Autodesk Inventor part; units mm, degrees
ref_plane "YZ Plane" through (0, 0, 0) normal (1, 0, 0) x (0, 1, 0)
ref_plane "XZ Plane" through (0, 0, 0) normal (0, 1, 0) x (-1, 0, 0)
ref_plane "XY Plane" through (0, 0, 0) normal (0, 0, 1) x (1, 0, 0)
sketch "Sketch1" plane through (0, 0, 0) normal (0, 1, 0) x (-1, 0, 0)
  line L0 (40.005, 40.005) -> (-40.005, 40.005)
  line L1 (-40.005, 40.005) -> (-40.005, -40.005)
  line L2 (-40.005, -40.005) -> (-33.3375, -40.005)
  line L3 (40.005, -40.005) -> (40.005, 40.005)
  line L4 (40.005, 40.005) -> (-40.005, -40.005) construction
  line L5 (-40.005, 40.005) -> (40.005, -40.005) construction
  line L6 (46.101, 46.101) -> (-46.101, 46.101)
  line L7 (-46.101, 46.101) -> (-46.101, -46.101)
  line L8 (-46.101, -46.101) -> (-33.3375, -46.101)
  line L9 (46.101, -46.101) -> (46.101, 46.101)
  line L10 (46.101, 46.101) -> (-46.101, -46.101) construction
  line L11 (-46.101, 46.101) -> (46.101, -46.101) construction
  line L12 (33.3375, -40.005) -> (33.3375, -46.101)
  line L13 (13.335, -40.005) -> (13.335, -46.101)
  line L14 (13.335, -40.005) -> (33.3375, -40.005)
  line L15 (33.3375, -46.101) -> (46.101, -46.101)
  line L16 (13.335, -46.101) -> (33.3375, -46.101)
  line L17 (33.3375, -40.005) -> (40.005, -40.005)
  line L18 (-20.9635, 41.5612) -> (22.9239, 41.5612) construction
  line L19 (22.9239, 41.5612) -> (22.9239, 28.3672) construction
  line L20 (22.9239, 28.3672) -> (-20.9635, 28.3672) construction
  line L21 (-20.9635, 28.3672) -> (-20.9635, 41.5612) construction
  line L22 (4.0005, -46.101) -> (4.0005, -40.005)
  line L23 (-4.0005, -46.101) -> (-4.0005, -40.005)
  line L24 (-13.335, -46.101) -> (-13.335, -40.005)
  line L25 (-33.3375, -46.101) -> (-33.3375, -40.005)
  line L26 (4.0005, -40.005) -> (13.335, -40.005)
  line L27 (-4.0005, -40.005) -> (4.0005, -40.005)
  line L28 (-4.0005, -46.101) -> (4.0005, -46.101)
  line L29 (4.0005, -46.101) -> (13.335, -46.101)
  line L30 (-13.335, -46.101) -> (-4.0005, -46.101)
  line L31 (-33.3375, -46.101) -> (-13.335, -46.101)
  line L32 (-33.3375, -40.005) -> (-13.335, -40.005)
  line L33 (-13.335, -40.005) -> (-4.0005, -40.005)
  point P0 (0, 0)
  dimension "baseLength" = 80.01
  dimension "d1" = 80.01
  dimension "d2" = 6.096
  dimension "toothLength" = 20.0025
  dimension "toothOffset" = 13.335
  dimension "d16" = 8.001
  dimension "d17" = 4.0005
  dimension "d18" = 20.0025
  dimension "d19" = 13.335
extrude "Extrusion1" add sketch "Sketch1" along normal blind 6.096 contours L3 L17 L14 L26 L27 L33 L32 L2 L1 L0
extrude "Extrusion2" add sketch "Sketch1" along normal blind 6.096 contours L12 L16 L13 L14 | L32 L24 L31 L25 | L22 L28 L23 L27
pattern_circular "Circular Pattern1" count 4 over 360 about axis through (0, -10, 0) along (0, 1, 0) of "Extrusion2"
equation "\"baseLength\" = glassLength"
equation "\"d1\" = baseLength"
equation "\"d2\" = woodThickness"
equation "\"toothLength\" = 0.25 * baseLength"
equation "\"d16\" = 0.4 * toothLength"
equation "\"d18\" = toothLength"
equation "\"d6\" = woodThickness"
equation "\"d8\" = woodThickness"
equation "\"woodThickness\" = 6.096"
equation "\"glassLength\" = 80.01"
equation "\"glassHeight\" = 80.772"
equation "\"lip\" = 9.525"
equation "\"lasorTol\" = 0.0635"
properties part number "CandleHolder-1"
Model file for the job. Use its own axes, mm. A direction names the side the tool comes from. Round coordinates to 2 decimals unless told otherwise and drop trailing zeros. Order: outer loops, then holes, each group sorted by start corner. A loop starts at its lowest first (then second) coordinate and runs counter-clockwise, first axis right, second up. Notation, with made-up numbers: (26.5, -2.5) -> (68.5, -2.5) arc R13 ccw to (68.5, 14.5) -> close; hole circle Ø8 at (22, 73). An arc over 180 degrees is marked (long way). Use one line per item in the form item = value.
Item 1: Cut at A-A, the plane z = 11. Write the cut outline in (x, y) (3 decimals).
Returned:
outline = (-40.005, 0) -> (40.005, 0) -> (40.005, 6.096) -> (-40.005, 6.096) -> close
Item 2: Tool access for faces 5 (the face through (43, 3, -13.335)), 6 (the face through (13.335, 3, -43)), 7 (the face through (37, 3, 40.005)): list every direction of +Z, -Z, +X, -X, +Y, -Y with a clear straight run to the whole face (end or side of a thin tool).
Returned:
face_5 = +X, +Y, -Y
face_6 = -Z, +Y, -Y
face_7 = +Z, +X, +Y, -Y
Item 3: Cut at B-B, the plane x = 37.5. Write the cut outline in (y, z) (3 decimals), and give its area (3 significant figures).
Returned:
outline = (0, -40.005) -> (6.096, -40.005) -> (6.096, 40.005) -> (0, 40.005) -> close
area = 488 mm^2
Item 4: Drill centre lines: line 1 (X direction, y = 4.75, z = 42.5) (1 decimal); line 2 (X direction, y = 2, z = 10.5) (3 decimals). Where is each one in solid material? Low to high.
Returned:
line_1 = -33.3 to -13.3, -4 to 4, 13.3 to 33.3
line_2 = -40.005 to 40.005
Item 5: Pull direction X, two halves, no side cores. Call faces 1 (the face through (33.338, 3, 43)), 2 (the face through (4, 3, 43)), 3 (the face through (4, 3, -43)), 4 (the face through (-43, 3, 4)): released by +X, released by -X, zero draft, split by the parting line, or undercut.
Returned:
face_1 = released by +X
face_2 = undercut
face_3 = undercut
face_4 = zero draft
Item 6: Flat gauge pins, fed straight in: pin 1 Ø1.8 at (y, z) = (3, -36) entering from -X (3 decimals); pin 2 Ø1.5 at (x, y) = (-12, 5) entering from +Z (3 decimals); pin 3 Ø1.8 at (y, z) = (2, -42.5) entering from +X; pin 4 Ø3 at (x, y) = (-5, 4.5) entering from -Z. Where does each tip first touch, or does it go through?
Returned:
pin_1 = -40.005
pin_2 = 40.005
pin_3 = 33.34
pin_4 = -46.1
